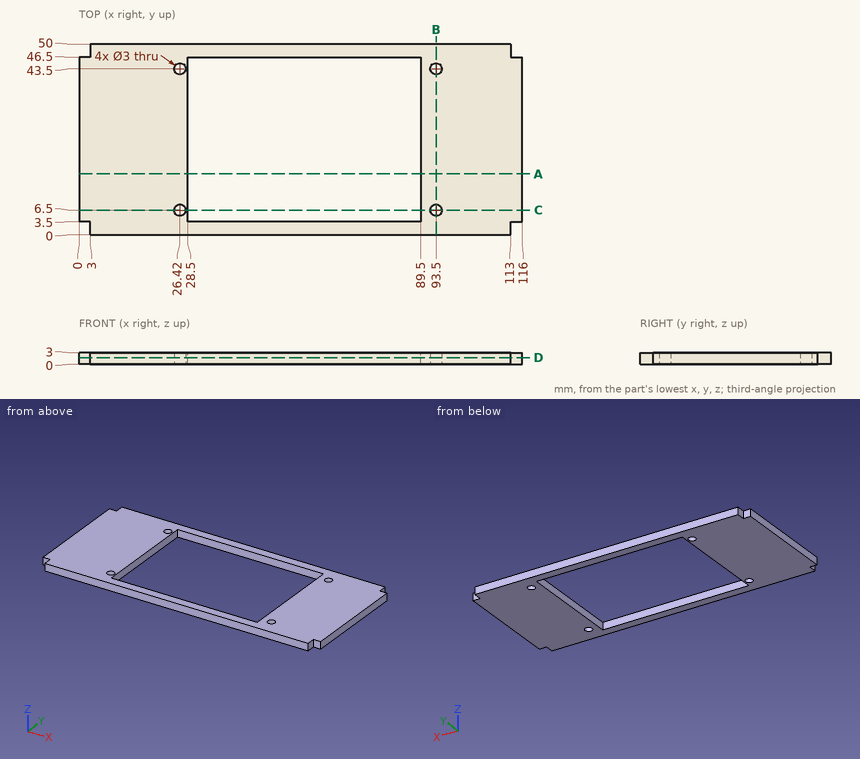
Geometry: see drawing. Coordinates: mm, zero at the bounding-box minimum. Give positions to 0.01 mm unless a question says otherwise; leave off trailing zeros. Order: outer loops, then holes, each group sorted by start corner. A loop starts at its lowest first (then second) coordinate and runs counter-clockwise, first axis right, second up.
1. Line query: probe 1 along Y at (x, z) = (26.42, 2.3); probe 2 along X at (y, z) = (6.5, 1.3); probe 3 along X at (y, z) = (22.5, 2.4). Output: solid intervals per line, ascending.
Computed:
probe 1: y = 0 to 5, 8 to 42, 45 to 50
probe 2: x = 0 to 24.92, 27.92 to 28.5, 89.5 to 92, 95 to 116
probe 3: x = 0 to 28.5, 89.5 to 116
2. Pin query (flat end, axial travel): pin 1 Ø0.9 at (y, z) = (1.5, 1.5) entering from +X; pin 2 Ø1.5 at (x, z) = (114.5, 1) entering from -Y; pin 3 Ø0.9 at (x, z) = (115, 1) entering from +Y. Return the tip coordinate at first contact, or that it passes through.
Computed:
pin 1: stops at x = 113
pin 2: stops at y = 3.5
pin 3: stops at y = 46.5
3. Cut plane C-C (y = 6.5). Return loops of the section in (x, z), and give its area (3 significant figures).
Computed:
outline: (0, 0) - (24.92, 0) - (24.92, 3) - (0, 3) - close; (27.92, 0) - (28.5, 0) - (28.5, 3) - (27.92, 3) - close; (89.5, 0) - (92, 0) - (92, 3) - (89.5, 3) - close; (95, 0) - (116, 0) - (116, 3) - (95, 3) - close
area: 147 mm2
4. Cut plane A-A (y = 16). Return loops of the section in (x, z), and give its area (3 significant figures).
Computed:
outline: (0, 0) - (28.5, 0) - (28.5, 3) - (0, 3) - close; (89.5, 0) - (116, 0) - (116, 3) - (89.5, 3) - close
area: 165 mm2
5. Cut plane B-B (x = 93.5). Return loops of the section in (y, z), and give its area (3 significant figures).
Computed:
outline: (0, 0) - (5, 0) - (5, 3) - (0, 3) - close; (8, 0) - (42, 0) - (42, 3) - (8, 3) - close; (45, 0) - (50, 0) - (50, 3) - (45, 3) - close
area: 132 mm2
6. Cut plane D-D (z = 1.8). Return loops of the section in (x, y).
Computed:
outline: (0, 3.5) - (3, 3.5) - (3, 0) - (113, 0) - (113, 3.5) - (116, 3.5) - (116, 46.5) - (113, 46.5) - (113, 50) - (3, 50) - (3, 46.5) - (0, 46.5) - close; hole circle Ø3 at (26.42, 6.5); hole circle Ø3 at (26.42, 43.5); hole (28.5, 3.5) - (89.5, 3.5) - (89.5, 46.5) - (28.5, 46.5) - close; hole circle Ø3 at (93.5, 6.5); hole circle Ø3 at (93.5, 43.5)
